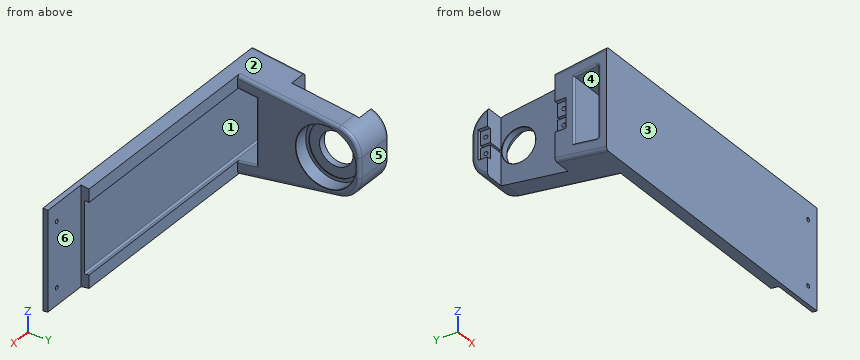
from build123d import *

# Parameters (mm, degrees)
SKETCH_1_W          = 190
SKETCH_1_H          = 60.00000000000001
EXTRUDE_1_DEPTH     = 8
EXTRUDE_2_DEPTH     = 76
SKETCH_3_W          = 29.999999999999986
SKETCH_3_H          = 60
CUT_EXTRUDE_1_DEPTH = 5
DRAFT_1_ANGLE       = 8.000000000000018
EXTRUDE_3_DEPTH     = 12
SKETCH_5_W          = 18.5
SKETCH_5_H          = 6.9999999999999964
CUT_EXTRUDE_2_DEPTH = 2.5
CUT_EXTRUDE_3_DEPTH = 211.0588577307207
SKETCH_7_R          = 18.750000000000007
CUT_EXTRUDE_4_DEPTH = 9
SKETCH_8_R          = 10.499999999999996
CUT_EXTRUDE_5_DEPTH = 195.81715456071922
SKETCH_10_R         = 16.750000000000007
CUT_EXTRUDE_7_DEPTH = 0.5
FILLET_2_R          = 15
FILLET_3_R          = 1
CHAMFER_1_SIZE      = 0.2
FILLET_4_R          = 2
SKETCH_9_R          = 1.2500000000000004
CUT_EXTRUDE_6_DEPTH = 10
SKETCH_11_R         = 1.2499999999999978
CUT_EXTRUDE_9_DEPTH = 129.66516135432758


with BuildPart() as part:
    # 스케치1 → 보스-돌출1 (new body)
    with BuildSketch(Plane(origin=(0, 0, 0), x_dir=(1, 0, 0), z_dir=(0, 1, 0))):
        Rectangle(SKETCH_1_W, SKETCH_1_H)
    extrude(amount=EXTRUDE_1_DEPTH)

    # 스케치2 → 보스-돌출2 (add)
    with BuildSketch(Plane(origin=(0, 8, 0), x_dir=(1, 0, 0), z_dir=(0, 1, 0))):
        Polygon((-68.99999999999997, -29.999999999999993), (-82.99999999999999, -29.999999999999996), (-82.99999999999997, 30), (-68.99999999999997, 30.000000000000004), align=None)
    extrude(amount=EXTRUDE_2_DEPTH)

    # 스케치3 → 컷-돌출1 (cut)
    with BuildSketch(Plane(origin=(0, 8, 0), x_dir=(1, 0, 0), z_dir=(0, 1, 0))):
        with Locations((80, 3.55e-15)):
            Rectangle(SKETCH_3_W, SKETCH_3_H)
    extrude(amount=-CUT_EXTRUDE_1_DEPTH, mode=Mode.SUBTRACT)

    # 구배1
    draft_1_faces = [part.faces().sort_by_distance(p)[0] for p in [
        (1.421e-14, 2.0774022239325727, -30),
        (1.421e-14, 2.0774022239325727, 30),
    ]]
    draft(draft_1_faces, Plane.ZX.offset(8), DRAFT_1_ANGLE)

    # 스케치4 → 보스-돌출3 (add)
    with BuildSketch(Plane.ZY.offset(82.99999999999997)):
        Polygon((-19.318896562618214, 83.99999999999999), (19.318896562618214, 83.99999999999999), (20.724304909642164, 74), (0.7500000000000067, 74), (0.7500000000000067, 80), (-0.7499999999999934, 80), (-0.7499999999999934, 74), (-20.724304909642132, 74), align=None)
        Polygon((0.7500000000000067, 32), (26.627019967142623, 32), (30.000000000000014, 8), (-29.999999999999986, 8), (-26.627019967142584, 32), (-0.7499999999999934, 32), (-0.7499999999999934, 25), (0.7500000000000067, 25), align=None)
    extrude(amount=EXTRUDE_3_DEPTH)

    # 스케치5 → 컷-돌출2 (cut)
    with BuildSketch(Plane.ZY.offset(94.99999999999999)):
        Polygon((-9.25, 80), (9.25, 80.00000000000001), (9.250000000000002, 74), (-9.249999999999998, 74), align=None)
        with Locations((-1.78e-15, 28.5)):
            Rectangle(SKETCH_5_W, SKETCH_5_H)
    extrude(amount=-CUT_EXTRUDE_2_DEPTH, mode=Mode.SUBTRACT)

    # 스케치6 → 컷-돌출3 (cut, through all)
    with BuildSketch(Plane.ZY.offset(94.99999999999999)):
        Polygon((-20.234889403422354, 20), (-22.34300192395823, 4.999999999999996), (22.343001923958226, 5.000000000000001), (20.23488940342236, 20), align=None)
    extrude(amount=-CUT_EXTRUDE_3_DEPTH, mode=Mode.SUBTRACT)

    # 스케치7 → 컷-돌출4 (cut)
    with BuildSketch(Plane(origin=(-68.99999999999997, 0, 0), x_dir=(0, 0, -1), z_dir=(1, 0, 0))):
        with Locations((2.22e-15, 62.9)):
            Circle(SKETCH_7_R)
    extrude(amount=-CUT_EXTRUDE_4_DEPTH, mode=Mode.SUBTRACT)

    # 스케치8 → 컷-돌출5 (cut, through all)
    with BuildSketch(Plane(origin=(-77.99999999999997, 0, 0), x_dir=(0, 0, -1), z_dir=(1, 0, 0))):
        with Locations((2.22e-15, 62.9)):
            Circle(SKETCH_8_R)
    extrude(amount=-CUT_EXTRUDE_5_DEPTH, mode=Mode.SUBTRACT)

    # 스케치10 → 컷-돌출7 (cut)
    with BuildSketch(Plane(origin=(-77.99999999999997, 0, 0), x_dir=(0, 0, -1), z_dir=(1, 0, 0))):
        with Locations((2.22e-15, 62.9)):
            Circle(SKETCH_10_R)
    extrude(amount=-CUT_EXTRUDE_7_DEPTH, mode=Mode.SUBTRACT)

    # 필렛2
    fillet_2_edges = [part.edges().sort_by_distance(p)[0] for p in [
        (-81.99999999999997, 84, -19.31889656261823),
        (-81.99999999999997, 84, 19.318896562618217),
    ]]
    fillet(fillet_2_edges, radius=FILLET_2_R)

    # 필렛3
    fillet_3_edges = [part.edges().sort_by_distance(p)[0] for p in [
        (-68.99999999999997, 20, 3.55e-15),
        (-68.99999999999997, 14, 21.078134411636704),
        (-14.999999999999986, 5.000000000000001, 22.343001923958226),
        (-68.99999999999997, 14, -21.078134411636704),
        (-14.999999999999986, 4.999999999999996, -22.34300192395823),
        (-94.99999999999999, 20, 3.55e-15),
        (-94.99999999999999, 12.499999999999998, -21.288945663690292),
        (-94.99999999999999, 4.999999999999998, -3.55e-15),
        (-94.99999999999999, 12.5, 21.288945663690292),
    ]]
    fillet(fillet_3_edges, radius=FILLET_3_R)

    # 모따기1
    chamfer_1_edges = [part.edges().sort_by_distance(p)[0] for p in [
        (-68.99999999999997, 62.9, 18.750000000000004),
        (-82.99999999999999, 62.9, 10.499999999999995),
    ]]
    chamfer(chamfer_1_edges, length=CHAMFER_1_SIZE)

    # 필렛4
    fillet_4_edges = [part.edges().sort_by_distance(p)[0] for p in [
        (-94.99999999999997, 83.99999999999999, -1.365e-14),
        (-68.99999999999997, 84, 0),
        (-68.99999999999997, 39.54379825720049, -25.566808263249197),
        (-68.99999999999997, 39.54379825720049, 25.566808263249193),
        (-68.99999999999999, 80.32064370334157, -16.120480930232446),
        (-68.99999999999999, 80.32064370334157, 16.120480930232446),
        (-94.99999999999999, 81.24744871391589, -14.93984953321921),
        (-94.99999999999999, 81.24744871391587, 14.939849533219187),
        (-94.99999999999997, 16, 28.87567332238087),
        (-94.99999999999999, 16, -28.875673322380862),
    ]]
    fillet(fillet_4_edges, radius=FILLET_4_R)

    # 스케치9 → 컷-돌출6 (cut)
    with BuildSketch(Plane.ZY.offset(92.49999999999999)):
        with Locations((-5.000000000000003, 76.75000000000001)):
            Circle(SKETCH_9_R)
        with Locations((4.999999999999997, 76.75)):
            Circle(SKETCH_9_R)
        with Locations((-4.9999999999999964, 28.150000000000002)):
            Circle(SKETCH_9_R)
        with Locations((5.000000000000004, 28.150000000000002)):
            Circle(SKETCH_9_R)
    extrude(amount=-CUT_EXTRUDE_6_DEPTH, mode=Mode.SUBTRACT)

    # 스케치11 → 컷-돌출9 (cut, through all)
    with BuildSketch(Plane(origin=(0, 3, 0), x_dir=(1, 0, 0), z_dir=(0, 1, 0))):
        with Locations(Location((87.00000000000003, 19.999999999999996, 0), (0, 0, 270))):
            Circle(SKETCH_11_R)
        with Locations(Location((87.00000000000003, -20.000000000000004, 0), (0, 0, 270))):
            Circle(SKETCH_11_R)
    extrude(amount=-CUT_EXTRUDE_9_DEPTH, mode=Mode.SUBTRACT)


solid = part.part
The listing builds one solid part. Answer for the finished solid, in the listing's coordinates (mm). Face numbers are marked on the shaded views. A direction names the side the tool comes from. Give positions to 0.01 mm unless a question says otherwise; leave off trailing zeros. Loops run counter-clockwise (first coordinate to the right, second up) from the corner with the lowest first, then second, coordinate; pieces in that order, holes last.
Item 1: Find the intervals of material crossed by line 1 along Y through (x, z) = (-88, 5); line 2 along Y through (x, z) = (-74, -5); line 3 along X through (y, z) = (1.75, -20), in increasing order.
Derived:
line 1: y = 0 to 5, 20 to 26.9, 29.4 to 32, 74 to 75.5, 78 to 84
line 2: y = 0 to 5, 20 to 44.83, 80.97 to 84
line 3: x = -95 to 85.75, 88.25 to 95
Item 2: A tool of negligible diameter and unlimited length cuts with its end or side. For the marked faces 4, 5 and 6, from which of +Z, -Z, +X, -X, +Y, -Y can it reach the whole face along a straight path? Write none if from no direction.
Derived:
face 4: +X, -X
face 5: +Z, -Z, +X, -X, +Y
face 6: +Z, -Z, +X, +Y
Item 3: Determine the mould class of the marked faces 1, 2 and 3 for opening direction Z: +Z half, -Z half, draft (parallel to the pull), parting line (faces both ways), or undercut.
Derived:
face 1: undercut
face 2: +Z half
face 3: draft
Item 4: Each of these flat-tipped pins is pushed along its axis until it touches: pin 1 Ø3 at (x, z) = (0, -19.5) entering from +Y; pin 2 Ø1.2 at (y, z) = (28.5, 4.5) entering from -X; pin 3 Ø2.5 at (y, z) = (76.75, 5) entering from +X; pin 4 Ø1.5 at (x, z) = (87, 20) entering from +Y. Where does it stop, or does it pass through?
Derived:
pin 1: stops at y = 5
pin 2: stops at x = -82.5
pin 3: stops at x = -78.5
pin 4: passes through
Item 5: A cutting plane is placed at A-A (x = 60.5). Give the vertices of the cut face in (y, z).
Derived:
outline: (0, -31.12) - (8, -30) - (8, -21.92) - (6.14, -22.18) arc R1 cw to (5, -21.19) - (5, 21.19) arc R1 cw to (6.14, 22.18) - (8, 21.92) - (8, 30) - (0, 31.12) - close
